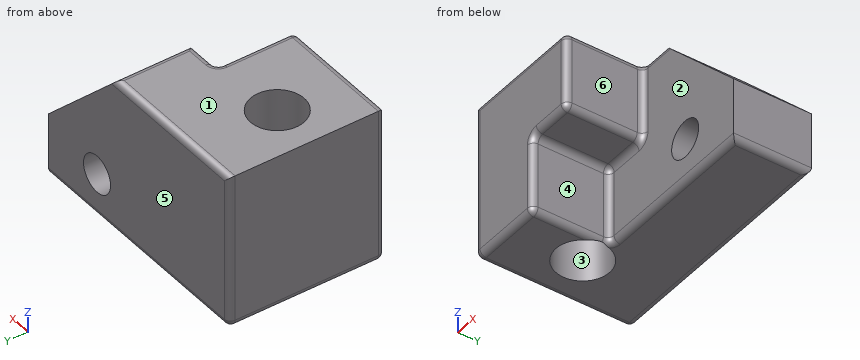
from build123d import *

# Parameters (mm, degrees)
F1_DEPTH = 127
F0_R     = 15.24
F2_DEPTH = 63.5
F3_SIZE  = 76.2
F4_R     = 5.08
F5_R     = 21.8454562642
F6_DEPTH = 228.6


with BuildPart() as f1:
    # F0 (on Front) → F1 (new body)
    with BuildSketch(Plane.XZ):
        Polygon((-26.7983935773, 0), (-26.7983935773, 63.5), (-128.3983935773, 63.5), (-128.3983935773, -63.5), (-64.8983935773, -63.5), (-64.8983935773, 0), align=None)
    extrude(amount=F1_DEPTH)

    # F0 (on Front) → F2 (join)
    with BuildSketch(Plane.XZ):
        Polygon((74.8016064227, -63.5), (74.8016064227, 63.5), (-26.7983935773, 63.5), (-26.7983935773, 0), (-64.8983935773, 0), (-64.8983935773, -63.5), align=None)
        with Locations((20.1709009707, -28.3607393503)):
            Circle(F0_R, mode=Mode.SUBTRACT)
    extrude(amount=F2_DEPTH)

    # F3
    f3_edges = [f1.edges().sort_by_distance(p)[0] for p in [
        (74.801606, -31.75, 63.5),
    ]]
    chamfer(f3_edges, length=F3_SIZE)

    # F4
    f4_edges = [f1.edges().sort_by_distance(p)[0] for p in [
        (-1.398394, -31.75, 63.5),
        (-128.398394, 0, 0),
        (-26.798394, -63.5, 31.75),
        (-45.848394, -63.5, 0),
        (-64.898394, -95.25, 0),
        (-26.798394, -95.25, 63.5),
        (-14.098394, -63.5, 63.5),
        (-64.898394, 0, 63.5),
        (-96.648394, -127, -63.5),
        (-128.398394, -127, 0),
        (-77.598394, -127, 63.5),
        (-64.898394, -95.25, -63.5),
        (-45.848394, -127, 0),
        (-64.898394, -127, -31.75),
        (-64.898394, -63.5, -31.75),
        (-128.398394, -63.5, -63.5),
        (-26.798394, -127, 31.75),
        (-26.798394, -95.25, 0),
        (74.801606, -31.75, -63.5),
        (-26.798394, 0, -63.5),
        (4.951606, -63.5, -63.5),
    ]]
    fillet(f4_edges, radius=F4_R)

    # F5 (on face) → F6 (cut)
    with BuildSketch(Plane.XY.offset(63.5)):
        with Locations((-88.2410332561, -68.5802102089)):
            Circle(F5_R)
    extrude(amount=-F6_DEPTH, mode=Mode.SUBTRACT)


solid = f1.part
Geometry: final body of the model. Coordinates: model frame, mm. Face numbers are marked on the shaded views. A direction names the side the tool comes from. Coordinates: 2 decimals unless noted, no trailing zeros. Order: outer loops, then holes, each group sorted by start corner. A loop starts at its lowest first (then second) coordinate and runs counter-clockwise, first axis right, second up.
(1) Material intervals for probe 1 along X at (y, z) = (-48.5, -42.5); probe 2 along Z at (x, y) = (8.5, -30.5); probe 3 along X at (y, z) = (-85.5, -35.5), sorted ascending.
(2) Section query A-A (x = -89). Return the cut outline in (y, z).
(3) Section query B-B (y = -7.5). Return the cut outline in (x, z).
(4) Access query for the marked faces 4, 5 and 6. Directions: +Z, -Z, +X, -X, +Y, -Y. A direction counts if a zero-diameter tool reaches every point of the face in a straight line with its end or side. Return the directions, or none.
(5) Section query C-C (z = 19). Return the cut outline in (x, y).
(6) Draft query along Y for the marked faces 1, 2 and 3. Return one class per face: pulls with the +Y half, pulls with the -Y half, needs draft (parallel to the pull), parting line crosses it, or undercut.
(7) First-contact query: pin 1 (2 mm diameter, centred on y = -107, z = 5.5, fed in from +X); pin 2 (4 mm diameter, centred on x = 42.5, y = -61.5, fed in from -Z); pin 3 (8.5 mm diameter, centred on x = -47, y = -94.5, fed in from -Z); pin 4 (24.5 mm diameter, centred on x = 20.17, z = -28.36, fed in from -Y). Flat tips, straight axial feed; report the tip coordinate or a pass-through.
(8) Section query D-D (x = -54). Return the cut outline in (y, z).
Solution:
1. probe 1: x = -128.4 to -96.84, -79.64 to 14.48, 25.86 to 74.8
1. probe 2: z = -63.5 to -38.16, -18.56 to 53.6
1. probe 3: x = -128.4 to -102.06, -74.42 to -64.9
2. outline: (-127, -58.42) arc R5.08 ccw to (-121.92, -63.5) - (-90.41, -63.5) - (-90.41, 63.5) - (-121.92, 63.5) arc R5.08 ccw to (-127, 58.42) - close; (-46.75, -63.5) - (-5.08, -63.5) arc R5.08 ccw to (0, -58.42) - (0, 58.42) arc R5.08 ccw to (-5.08, 63.5) - (-46.75, 63.5) - close
3. outline: (-128.4, -58.42) arc R5.08 ccw to (-123.32, -63.5) - (69.72, -63.5) arc R5.08 ccw to (74.8, -58.42) - (74.8, -12.7) - (0.09, 62.01) arc R5.08 ccw to (-3.5, 63.5) - (-128.4, 63.5) - close; hole circle Ø30.48 at (20.17, -28.36)
4. face 4: -Z, +X, -Y
4. face 5: +Z, -Z, +X, -X, +Y
4. face 6: +Z, -Z, +X, -Y
5. outline: (-128.4, -121.92) arc R5.08 ccw to (-123.32, -127) - (-31.88, -127) arc R5.08 ccw to (-26.8, -121.92) - (-26.8, -68.58) arc R5.08 cw to (-21.72, -63.5) - (43.1, -63.5) - (43.1, 0) - (-123.32, 0) arc R5.08 ccw to (-128.4, -5.08) - close; hole circle Ø43.69 at (-88.24, -68.58)
6. face 1: needs draft
6. face 2: pulls with the -Y half
6. face 3: undercut
7. pin 1: stops at x = -26.8
7. pin 2: stops at z = -63.38
7. pin 3: stops at z = 0
7. pin 4: passes through
8. outline: (-127, 5.08) arc R5.08 ccw to (-121.92, 0) - (-68.58, 0) arc R5.08 cw to (-63.5, -5.08) - (-63.5, -58.42) arc R5.08 ccw to (-58.42, -63.5) - (-5.08, -63.5) arc R5.08 ccw to (0, -58.42) - (0, 58.42) arc R5.08 ccw to (-5.08, 63.5) - (-121.92, 63.5) arc R5.08 ccw to (-127, 58.42) - close
